Job drawing, mm, ordinate dimensions from the low corner. One solid piece. Give positions to 0.01 mm unless a question says otherwise; leave off trailing zeros. Write each loop counter-clockwise with the first axis right and the second up, starting at its lowest first coordinate (ties: lowest second). Pieces come first, ordered by that corner, then holes. Notation, with made-up numbers: (60.5, 58) - (71.5, 58) arc R19 ccw to (71.5, 85) - close; hole circle Ø1 at (54, 59). An arc over 180 degrees is marked (long way). Put each result on its own line as item: value. Start each with the question number.
1. Drop flat-ended pins along their axis: pin 1 (1.6 mm diameter, centred on x = 38.5, y = 2, fed in from -Z); pin 2 (1 mm diameter, centred on y = 2, z = 79, fed in from -X). Give the stop position or say it passes through.
2. Cut at B-B on z = 25.4. List the corners of the cut face in (x, y) (1 decimal).
3. Cut at A-A on x = 85. List the corners of the cut face in (y, z) (1 decimal).
4. Cut at C-C on y = 0.75. Give the number of separate pieces and of enclosed holes in the cut face.
5. Cut at D-D on z = 60.5. List the corners of the cut face in (x, y) (1 decimal).
6. Wall check: line 1 (X direction, y = 2.8, z = 83) (1 decimal); line 2 (X direction, y = 0.2, z = 77) (1 decimal); line 3 (Z direction, x = 41.5, y = 2.1). Give the ranges that are in metal, low to high.
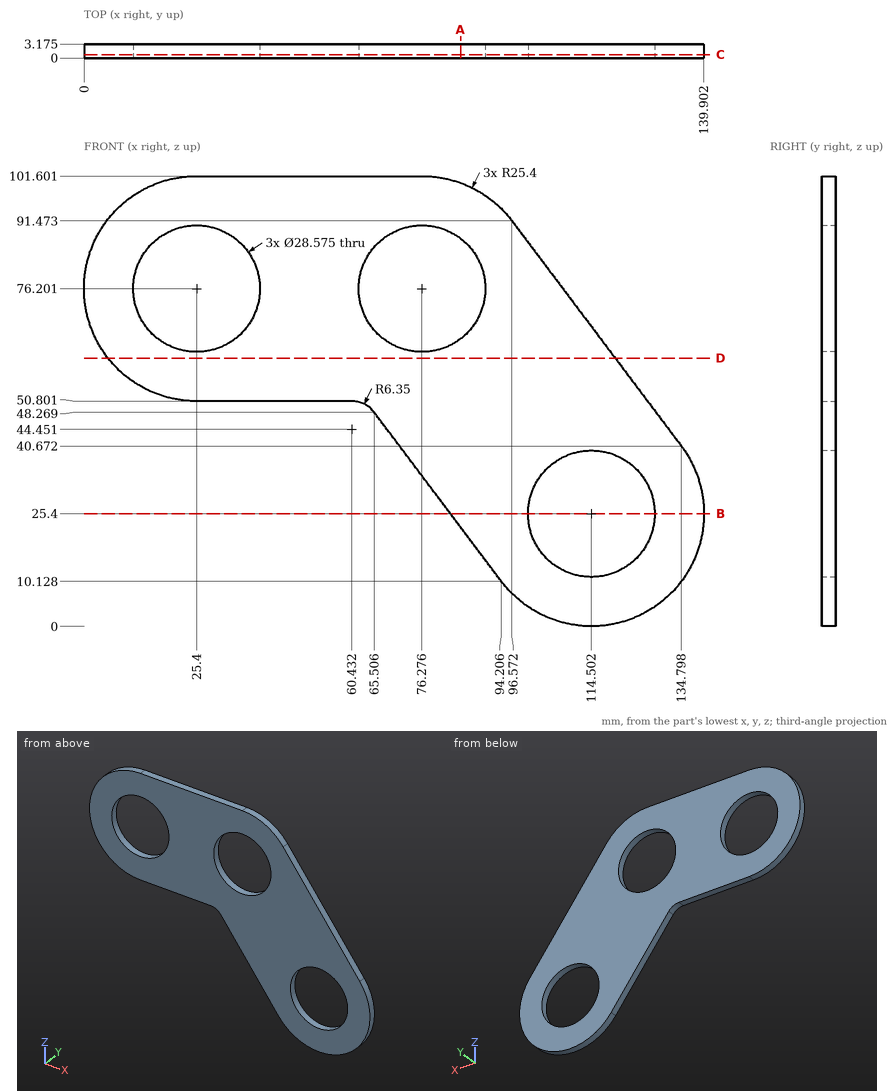
Report:
1. pin 1: stops at z = 50.8
1. pin 2: stops at x = 0.1
2. outline: (82.7, 0) - (100.2, 0) - (100.2, 3.2) - (82.7, 3.2) - close; (128.8, 0) - (139.9, 0) - (139.9, 3.2) - (128.8, 3.2) - close
3. outline: (0, 22.4) - (3.2, 22.4) - (3.2, 64.9) - (0, 64.9) - close; (0, 87.5) - (3.2, 87.5) - (3.2, 100.1) - (0, 100.1) - close
4. separate pieces: 1
4. enclosed holes: 3
5. outline: (5.4, 0) - (119.9, 0) - (119.9, 3.2) - (5.4, 3.2) - close
6. line 1: x = 0.9 to 12.8, 38 to 63.7, 88.8 to 102.9
6. line 2: x = 0 to 11.1, 39.7 to 62, 90.5 to 107.5
6. line 3: z = 50.8 to 101.6
